Check sheet for the modelled part. Datum: model origin and axes. Units: mm. Face numbers are marked on the shaded views. Coordinates: 2 decimals unless noted, no trailing zeros. Write each loop counter-clockwise with the first axis right and the second up, starting at its lowest first coordinate (ties: lowest second). Pieces come first, ordered by that corner, then holes. Notation, with made-up numbers: (60.5, -12.75) -> (114.5, -12.75) arc R15 ccw to (114.5, 10.25) -> close; hole circle Ø11 at (11.5, -2.5). An arc over 180 degrees is marked (long way). Put each result on its own line as item: value.
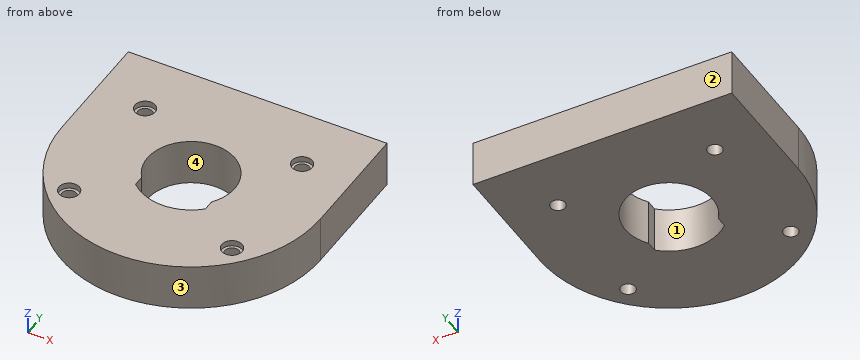
```python
from build123d import *

# Parameters (mm, degrees)
F0_R     = 2.5
F1_DEPTH = 16
F2_R     = 3.5
F3_DEPTH = 2


with BuildPart() as f1:
    # F0 (on Top) → F1 (new body)
    with BuildSketch(Plane.XY):
        with BuildLine():
            Line((44.5, 41), (-44.5, 41))
            Line((-44.5, 41), (-44.5, 0))
            ThreePointArc((-44.5, 0), (0, -44.5), (44.5, 0))
            Line((44.5, 0), (44.5, 41))
        make_face()
        with Locations((-28, -25)):
            Circle(F0_R, mode=Mode.SUBTRACT)
        with Locations((28, -25)):
            Circle(F0_R, mode=Mode.SUBTRACT)
        with Locations((-27, 20)):
            Circle(F0_R, mode=Mode.SUBTRACT)
        with BuildLine():
            ThreePointArc((-12, -9), (0, 15), (12, -9))
            Line((12, -9), (12, -12.737739))
            ThreePointArc((12, -12.737739), (0, -17.5), (-12, -12.737739))
            Line((-12, -12.737739), (-12, -9))
        make_face(mode=Mode.SUBTRACT)
        with Locations((27, 20)):
            Circle(F0_R, mode=Mode.SUBTRACT)
    extrude(amount=F1_DEPTH)

    # F2 (on face) → F3 (cut)
    with BuildSketch(Plane.XY.offset(16)):
        with Locations((-27, 20)):
            Circle(F2_R)
        with Locations((-28, -25)):
            Circle(F2_R)
        with Locations((27, 20)):
            Circle(F2_R)
        with Locations((28, -25)):
            Circle(F2_R)
    extrude(amount=-F3_DEPTH, mode=Mode.SUBTRACT)


solid = f1.part
```
Q1. Cross-section at C-C (z = 10.5). Record the cut outline in (x, y).
Recorded:
outline: (-44.5, 0) arc R44.5 ccw to (44.5, 0) -> (44.5, 41) -> (-44.5, 41) -> close; hole circle Ø5 at (-28, -25); hole circle Ø5 at (-27, 20); hole (-12, -12.74) arc R17.5 ccw to (12, -12.74) -> (12, -9) arc R15 ccw (long way) to (-12, -9) -> close; hole circle Ø5 at (27, 20); hole circle Ø5 at (28, -25)
Q2. Cross-section at A-A (x = 0). Record the cut outline in (y, z).
Recorded:
outline: (-44.5, 0) -> (-17.5, 0) -> (-17.5, 16) -> (-44.5, 16) -> close; (15, 0) -> (41, 0) -> (41, 16) -> (15, 16) -> close
Q3. Mould release check, pull along Y, two halves, no side actions. Record for the marked faces 1, 2, 3 and 4: released by +Y, released by -Y, zero draft, split by the parting line, or undercut.
Recorded:
face 1: undercut
face 2: released by +Y
face 3: released by -Y
face 4: undercut
Q4. Cross-section at D-D (x = -27). Record the cut outline in (y, z), plus the area to 3 significant figures.
Recorded:
outline: (-35.37, 0) -> (-27.29, 0) -> (-27.29, 14) -> (-28.35, 14) -> (-28.35, 16) -> (-35.37, 16) -> close; (-22.71, 0) -> (17.5, 0) -> (17.5, 14) -> (16.5, 14) -> (16.5, 16) -> (-21.65, 16) -> (-21.65, 14) -> (-22.71, 14) -> close; (22.5, 0) -> (41, 0) -> (41, 16) -> (23.5, 16) -> (23.5, 14) -> (22.5, 14) -> close
area: 1,060 mm2
Q5. Material ranges on line 1 along Y through (x, z) = (-27, 15.1); line 2 along X through (y, z) = (-25, 9.75); line 3 along Y through (x, z) = (-27, 8.25), recorded low to high.
Recorded:
line 1: y = -35.37 to -28.35, -21.65 to 16.5, 23.5 to 41
line 2: x = -36.81 to -30.5, -25.5 to 25.5, 30.5 to 36.81
line 3: y = -35.37 to -27.29, -22.71 to 17.5, 22.5 to 41
Q6. Depth check by flat-ended pin: P1, Ø6, axis at x = 7.5, z = 7, coming from the -Y side; P2, Ø3, axis at y = -10.5, z = 8, coming from the +X side; P3, Ø2, axis at x = -10.5, z = 8, coming from the -Y side. Enter the tip coordinate at first touch or a pass-through.
Recorded:
P1: stops at y = -44.27
P2: stops at x = 43.58
P3: stops at y = -43.47
Q7. Cross-section at B-B (y = 20). Record the cut outline in (x, z).
Recorded:
outline: (-44.5, 0) -> (-29.5, 0) -> (-29.5, 14) -> (-30.5, 14) -> (-30.5, 16) -> (-44.5, 16) -> close; (-24.5, 0) -> (24.5, 0) -> (24.5, 14) -> (23.5, 14) -> (23.5, 16) -> (-23.5, 16) -> (-23.5, 14) -> (-24.5, 14) -> close; (29.5, 0) -> (44.5, 0) -> (44.5, 16) -> (30.5, 16) -> (30.5, 14) -> (29.5, 14) -> close
